```python
from build123d import *

# Parameters (mm, degrees)
F0_W      = 270.002
F0_H      = 549.91
F1_DEPTH  = 25.4
F2_W      = 270.002
F2_H      = 549.91
F3_DEPTH  = 919.48
F4_T      = -20.32
F5_START  = 228.6
F4_FACE_W = 509.27
F4_FACE_H = 904.24
F5_DEPTH  = 20.32
F7_DEPTH  = 25.4
F8_R      = 152.4
F9_DEPTH  = 25.4
F10_R     = 54.61
F11_DEPTH = 25.4
F12_R     = 54.61
F13_DEPTH = 25.4
F14_W     = 120
F14_H     = 250
F15_DEPTH = 22
F16_DEPTH = 55.88
F17_W     = 120
F17_H     = 250
F18_DEPTH = 50.8


with BuildPart() as f1:
    # F0 (on Top) → F1 (new body)
    with BuildSketch(Plane.XY):
        Rectangle(F0_W, F0_H)
    extrude(amount=F1_DEPTH)

    # F2 (on face) → F3 (join)
    with BuildSketch(Plane.XY.offset(25.4)):
        Rectangle(F2_W, F2_H)
    extrude(amount=F3_DEPTH)

    # F4
    f4_openings = [f1.faces().sort_by_distance(p)[0] for p in [
        (135.001, 0, 472.44),
    ]]
    offset(amount=F4_T, openings=f4_openings)

    # F4_face (on face) → F5 (join)
    with BuildSketch(Plane(origin=(-114.681, 0, 472.44), x_dir=(0, 1, 0), z_dir=(1, 0, 0)).offset(F5_START)):
        Rectangle(F4_FACE_W, F4_FACE_H)
    extrude(amount=F5_DEPTH)

    # F6 (on face) → F7 (cut)
    with BuildSketch(Plane.YZ.offset(134.239)):
        with BuildLine():
            ThreePointArc((0, 843.28), (-107.7630734528, 583.1169265472), (152.4, 690.88))
            ThreePointArc((152.4, 690.88), (107.7630734528, 798.6430734528), (0, 843.28))
        make_face()
    extrude(amount=-F7_DEPTH, mode=Mode.SUBTRACT)

    # F8 (on face) → F9 (cut)
    with BuildSketch(Plane.YZ.offset(134.239)):
        with Locations((0, 304.8)):
            Circle(F8_R)
    extrude(amount=-F9_DEPTH, mode=Mode.SUBTRACT)

    # F10 (on face) → F11 (cut)
    with BuildSketch(Plane.YZ.offset(134.239)):
        with Locations((-169.545, 105.41)):
            Circle(F10_R)
    extrude(amount=-F11_DEPTH, mode=Mode.SUBTRACT)

    # F12 (on face) → F13 (cut)
    with BuildSketch(Plane.YZ.offset(134.239)):
        with Locations((169.545, 105.41)):
            Circle(F12_R)
    extrude(amount=-F13_DEPTH, mode=Mode.SUBTRACT)

    # F14 (on face) → F15 (join)
    with BuildSketch(Plane.XZ.offset(274.955)):
        with Locations((-0.001, 669.88)):
            Rectangle(F14_W, F14_H)
    extrude(amount=-F15_DEPTH)

    # F14 (on face) → F16 (cut)
    with BuildSketch(Plane.XZ.offset(274.955)):
        with Locations((-0.001, 669.88)):
            Rectangle(F14_W, F14_H)
    extrude(amount=-F16_DEPTH, mode=Mode.SUBTRACT)

    # F17 (on face) → F18 (cut)
    with BuildSketch(Plane(origin=(0, 274.955, 0), x_dir=(-1, 0, 0), z_dir=(0, 1, 0))):
        with Locations((0.001, 669.88)):
            Rectangle(F17_W, F17_H)
    extrude(amount=-F18_DEPTH, mode=Mode.SUBTRACT)


solid = f1.part
```
Verification items for the finished model (mm, model axes). A direction names the side the tool comes from. Round coordinates to 2 decimals unless told otherwise and drop trailing zeros. Write each loop counter-clockwise with the first axis right and the second up, starting at its lowest first coordinate (ties: lowest second). Pieces come first, ordered by that corner, then holes.
1. Section check A-A on x = 45. Enter the section's corners in (y, z) (3 decimals), plus the area to 3 significant figures.
2. Gauge pin test, flat ends, axial feed: P1, Ø1, axis at x = 93, y = -8.5, coming from the -Z side; P2, Ø12, axis at y = -5.5, z = 133, coming from the +X side. Record the tip position at first contact, or that the pin passes through.
3. Draft check along Y on faces 6 (the flat face through (-1, -265, 794.88)), 7 (the flat face through (113.919, -4, 479)), 8 (the flat face through (-2, 274.955, 466)), 9 (the flat face through (-2, 254.635, 466)). Enter one of: +Y half, -Y half, draft (parallel to the pull), parting line (faces both ways), or undercut.
4. Access from +Z, -Z, +X, -X, +Y, -Y to the whole of each face (thin tool, end or side, straight path). Record for faces 1 (the flat face through (-1, -265, 544.88)), 2 (the flat face through (135.001, -266, 470)), 3 (the flat face through (-2, 4, 20.32)), 4 (the cylindrical face through (124.221, -19.839, 841.983)), 5 (the flat face through (-135.001, -4, 466)).
5. Section check B-B on y = 0. Enter the section's corners in (x, z), plus the area to 3 significant figures.
6. Scan lines: L1, parallel to Z at x = 119, y = 0; L2, parallel to Z at x = -63, y = -48; L3, parallel to X at y = 133, z = 432.5. Record each from-to range of solid material in increasing order.
7. Section check D-D on x = -75. Enter the section's corners in (y, z) (3 decimals), plus the area to 3 significant figures.
8. Section check C-C on z = 690.88. Enter the section's corners in (x, y) (3 decimals), plus the area to 3 significant figures.
Answer:
1. outline: (-274.955, 0) - (274.955, 0) - (274.955, 544.88) - (254.635, 544.88) - (254.635, 20.32) - (-254.635, 20.32) - (-254.635, 544.88) - (-274.955, 544.88) - close; (-274.955, 794.88) - (-254.635, 794.88) - (-254.635, 924.56) - (254.635, 924.56) - (254.635, 794.88) - (274.955, 794.88) - (274.955, 944.88) - (-274.955, 944.88) - close
1. area: 48,900 mm2
2. P1: stops at z = 0
2. P2: stops at x = 134.24
3. face 6: draft
3. face 7: undercut
3. face 8: +Y half
3. face 9: undercut
4. face 1: +Y, -Y
4. face 2: +Z, -Z, +X, +Y, -Y
4. face 3: none
4. face 4: +X
4. face 5: +Z, -Z, -X, +Y, -Y
5. outline: (-135, 0) - (135, 0) - (135, 20.32) - (134.24, 20.32) - (134.24, 152.4) - (113.92, 152.4) - (113.92, 20.32) - (-114.68, 20.32) - (-114.68, 924.56) - (113.92, 924.56) - (113.92, 843.28) - (134.24, 843.28) - (134.24, 924.56) - (135, 924.56) - (135, 944.88) - (-135, 944.88) - close; (113.92, 457.2) - (134.24, 457.2) - (134.24, 538.48) - (113.92, 538.48) - close
5. area: 35,300 mm2
6. L1: z = 0 to 152.4, 457.2 to 538.48, 843.28 to 944.88
6. L2: z = 0 to 20.32, 924.56 to 944.88
6. L3: x = -135 to -114.68, 113.92 to 134.24
7. outline: (-274.955, 0) - (274.955, 0) - (274.955, 944.88) - (-274.955, 944.88) - close; hole (-254.635, 20.32) - (254.635, 20.32) - (254.635, 924.56) - (-254.635, 924.56) - close
7. area: 59,100 mm2
8. outline: (-135.001, -274.955) - (-60.001, -274.955) - (-60.001, -254.635) - (-114.681, -254.635) - (-114.681, 254.635) - (-60.001, 254.635) - (-60.001, 274.955) - (-135.001, 274.955) - close; (59.999, -274.955) - (135.001, -274.955) - (135.001, -254.635) - (134.239, -254.635) - (134.239, -152.4) - (113.919, -152.4) - (113.919, -254.635) - (59.999, -254.635) - close; (59.999, 254.635) - (113.919, 254.635) - (113.919, 152.4) - (134.239, 152.4) - (134.239, 254.635) - (135.001, 254.635) - (135.001, 274.955) - (59.999, 274.955) - close
8. area: 20,600 mm2
